Autodesk Inventor part; units mm, degrees
ref_plane "Work Plane1" through (0, 0, -7) normal (0, 0, -1) x (-1, 0, 0)
ref_plane "YZ Plane" through (0, 0, 0) normal (1, 0, 0) x (0, 1, 0)
ref_plane "XZ Plane" through (0, 0, 0) normal (0, 1, 0) x (-1, 0, 0)
sketch "Sketch1" plane through (0, 0, 0) normal (0, 0, 1) x (1, 0, 0)
  circle A0 centre (0, 0) radius 2.5
  circle A1 centre (20, 0) radius 2.5
  line L0 (7, 10) -> (20, 10)
  line L1 (7, -10) -> (20, -10)
  arc A2 (20, -10) -> (20, 10) centre (20, 0) ccw
  line L2 (7, 10) -> (7, 8)
  line L3 (7, -10) -> (7, -8)
  line L4 (7, 8) -> (0, 8)
  line L5 (7, -8) -> (0, -8)
  arc A3 (0, 8) -> (0, -8) centre (0, 0) ccw
  dimension "d0" = 5
  dimension "d1" = 20
  dimension "d2" = 10
  dimension "d3" = 2
  dimension "d4" = 13
extrude "Extrusion1" add sketch "Sketch1" along normal blind 4
sketch "Sketch2" plane through (0, 0, 4) normal (0, 0, 1) x (1, 0, 0)
  circle A0 centre (0, 0) radius 2.5
  line L0 (7, 8) -> (0, 8)
  arc A1 (0, 8) -> (0, -8) centre (0, 0) ccw
  line L1 (0, -8) -> (7, -8)
  line L2 (7, -10) -> (20, -10)
  line L3 (7, 8) -> (7, -8)
  line L4 (7, -8) -> (0, -8)
  line L5 (7, 8) -> (0, 8)
  arc A2 (0, 8) -> (0, -8) centre (0, 0) ccw
extrude "Extrusion2" cut sketch "Sketch2" against normal blind 2
sketch "Sketch3" plane through (0, 0, 0) normal (0, 0, -1) x (-1, 0, 0)
  circle A0 centre (-20, 0) radius 2.5
  circle A1 centre (0, 0) radius 2.5
  line L0 (-7, 10) -> (-20, 10)
  arc A2 (-20, 10) -> (-20, -10) centre (-20, 0) ccw
  line L1 (-20, -10) -> (-7, -10)
  line L2 (-7, 8) -> (-7, 10)
  line L3 (-19, 10) -> (-19, 8)
  line L4 (-19, 8) -> (-11, 8)
  line L5 (-11, 8) -> (-11, -8)
  line L6 (-11, -8) -> (-19, -8)
  line L7 (-19, -8) -> (-19, -10)
  point P0 (-7, -8)
  dimension "d9" = 1
  dimension "d10" = 11
extrude "Extrusion3" cut sketch "Sketch3" against normal blind 2 contours L3 L4 L5 L6 L7 L1 A2 L0
sketch "Sketch4" plane through (0, 0, 4) normal (0, 0, 1) x (1, 0, 0)
  line L0 (7, 10) -> (7, -10)
  circle A0 centre (0, 0) radius 2.5
  arc A1 (7, -8.4853) -> (7, 8.4853) centre (0, 0) ccw
  dimension "d15" = 11
extrude "Extrusion4" cut sketch "Sketch4" against normal blind 2 contours A1 L0
sketch "Sketch5" plane through (0, 0, 0) normal (0, 0, -1) x (-1, 0, 0)
  line L0 (0, 8) -> (-7, 8)
  line L1 (-7, 10) -> (0, 10)
  line L2 (0, 10) -> (0, 8)
  line L3 (0, 8) -> (-7, 8)
  line L4 (-7, 8) -> (-7, 10)
  arc A0 (0, -8) -> (0, 8) centre (0, 0) ccw
extrude "Extrusion5" add sketch "Sketch5" against normal blind 2
sketch "Sketch6" plane through (0, 0, 0) normal (0, 0, -1) x (-1, 0, 0)
  line L0 (0, 10) -> (-19, 10)
  line L1 (-19, 8) -> (-20, 8)
  line L2 (-20, 8) -> (-20, 10)
  line L3 (-20, 10) -> (-19, 10)
  line L4 (-19, 10) -> (-19, 8)
  circle A0 centre (-20, 0) radius 2.5
extrude "Extrusion6" add sketch "Sketch6" against normal blind 2 contours L1 L2 L3 L4
sketch "Sketch7" plane through (0, 0, 0) normal (0, 0, -1) x (-1, 0, 0)
  line L0 (-19, -8) -> (-19, -10)
  line L1 (-11, -8) -> (-19, -8)
  line L2 (-17.4006, -8) -> (-19, -9.162)
  line L3 (-17.4006, -8) -> (-26.8052, 4.9443) construction
  line L4 (-26.8052, 4.9443) -> (-28.4046, 3.7823) construction
  line L5 (-28.4046, 3.7823) -> (-19, -9.162) construction
  circle A0 centre (-20, 0) radius 2.5
  line L6 (-17.4006, -8) -> (-19, -8)
  line L7 (-19, -8) -> (-19, -9.162)
  dimension "d21" = 16
  dimension "d22" = 8
  dimension "d23" = 36
extrude "Extrusion7" cut sketch "Sketch7" against normal blind 2 contours L1 L2 L0
sketch "Sketch9" plane through (0, 0, 2) normal (0, 0, 1) x (1, 0, 0)
  circle A0 centre (0, 0) radius 2.5
  arc A1 (11, 0) -> (7, 8.4853) centre (0, 0) ccw
  circle A2 centre (0, 0) radius 2.5
extrude "Extrusion8" add sketch "Sketch9" along normal mid plane 4
fillet "Fillet1" radius 0.5 1 edges at (-2.5, 0, 4)
sketch "Sketch10" plane through (0, 0, 0) normal (0, 0, -1) x (-1, 0, 0)
  arc A0 (0, -8) -> (0, 8) centre (0, 0) ccw
  line L0 (0, 10) -> (-20, 10)
  line L1 (4.7023, 6.4721) -> (11.1744, 1.7699)
  line L2 (11.1744, 1.7699) -> (6.4721, -4.7023)
  dimension "d30" = 144
extrude "Extrusion9" add sketch "Sketch10" against normal blind 2
fillet "Fillet2" radius 6 1 edges at (-11.1744, 1.7699, 1)
ref_plane "Work Plane1" through (0, 0, -7) normal (0, 0, -1) x (-1, 0, 0)
mirror "Mirror1" about plane through (0, 0, -7) normal (0, 0, -1)
sketch "Sketch11" plane through (0, 0, 0) normal (0, 0, -1) x (-1, 0, 0)
  arc A0 (4.7023, 6.4721) -> (0, 8) centre (0, 0) ccw
  line L0 (0, 8) -> (0, 10)
  line L1 (0, 10) -> (-20, 10)
  line L2 (-20, 10) -> (-20, 8)
  line L3 (-20, 8) -> (-11, 8)
  line L4 (-11, -8) -> (-17.4006, -8)
  line L5 (-17.4006, -8) -> (-19, -9.162)
  line L6 (-19, -9.162) -> (-19, -10)
  line L7 (-19, -10) -> (-7, -10)
  line L8 (-7, -10) -> (-7, -8)
  line L9 (-7, -8) -> (0, -8)
  line L10 (-11, -8) -> (-7, -8)
  line L11 (-11, 8) -> (0, 8)
extrude "Extrusion10" add sketch "Sketch11" along normal blind 14
properties part number "cable_chain_22" material "ABS Plastic"
Source: CAD feature listing. Evaluate the final solid. Frame: model axes, mm. A direction names the side the tool comes from. Coordinates: 2 decimals unless noted, no trailing zeros. Loops run counter-clockwise (first coordinate to the right, second up) from the corner with the lowest first, then second, coordinate; pieces in that order, holes last. Notation, with made-up numbers: (31.5, 34) -> (38.5, 34) arc R28 cw to (38.5, 70) -> close; hole circle Ø11 at (32.25, 44.5). An arc over 180 degrees is marked (long way). Answer in a Markdown table with one row per item. Add a question column.
Q1. Ray query, line 1 along Y through (x, z) = (12.5, -5.5); line 2 along Y through (x, z) = (20, 2.5); line 3 along Z through (x, y) = (17, 3.25). Return the intervals inside material, ascending.
Q2. Section B-B on z = -12. Return the cut outline in (x, y), and give its area (3 significant figures).
Q3. Section A-A on z = 2.75. Return the cut outline in (x, y).
Q4. Pull-direction query (Z, two-part tool) for faces 6 (the face through (10, 8, -7)), 7 (the face through (18.189, -8.573, -6.874)), 8 (the face through (10, 10, -7)), 9 (the face through (3, 1, 2)); classes: pulls with the +Z half, pulls with the -Z half, needs draft (parallel to the pull), parting line crosses it, or undercut.
Q5. Section C-C on x = 22. Return the cut outline in (y, z), and give its area (3 significant figures).
Q6. Contact query for flat-ended pins moving along their axis: pin 1 Ø6 at (x, y) = (9.5, 4.5) entering from -Z; pin 2 Ø1.6 at (x, z) = (3.5, 0.5) entering from -Y; pin 3 Ø1.7 at (y, z) = (9, -17) entering from -X; pin 4 Ø1.6 at (y, z) = (9.5, -4.5) entering from +X. Output: stop coordinate, or through.
Q7. Reachability of faces 1 (the face through (11, 0, -15)), 2 (the face through (1, 0, -14)), 3 (the face through (-5.5, 5.893, 0.986)), 4 (the face through (7, 9, 3)), 5 (the face through (3, 1, -16)) from +Z, -Z, +X, -X, +Y, -Y: full face, straight path, thin tool, end or side. Return the list, or none.
Q8. Section D-D on y = -6.5. Return the cut outline in (x, z), and give its area (3 significant figures).
Computed values:
| question | item | result |
|---|---|---|
| 1 | line 1 | y = -10 to -8, 8 to 10 |
| 1 | line 2 | y = -10 to -2.5, 2.5 to 10 |
| 1 | line 3 | z = -18 to -16, 2 to 4 |
| 2 | outline | (0, 8) -> (20, 8) -> (20, 10) -> (0, 10) -> close; (7, -10) -> (19, -10) -> (19, -9.16) -> (17.4, -8) -> (7, -8) -> close |
| 2 | area | 63.1 mm^2 |
| 3 | outline | circle Ø5 at (0, 0); (7, -10) -> (20, -10) arc R10 ccw to (20, 10) -> (7, 10) -> (7, 8.49) arc R11 cw to (7, -8.49) -> close; hole circle Ø5 at (20, 0) |
| 4 | face 6 | undercut |
| 4 | face 7 | undercut |
| 4 | face 8 | needs draft |
| 4 | face 9 | pulls with the +Z half |
| 5 | outline | (-9.8, -18) -> (-1.5, -18) -> (-1.5, -16) -> (-9.8, -16) -> close; (-9.8, 2) -> (-1.5, 2) -> (-1.5, 4) -> (-9.8, 4) -> close; (1.5, -18) -> (9.8, -18) -> (9.8, -16) -> (1.5, -16) -> close; (1.5, 2) -> (9.8, 2) -> (9.8, 4) -> (1.5, 4) -> close |
| 5 | area | 66.4 mm^2 |
| 6 | pin 1 | stops at z = -18 |
| 6 | pin 2 | stops at y = -8 |
| 6 | pin 3 | stops at x = 7 |
| 6 | pin 4 | stops at x = 20 |
| 7 | face 1 | +X |
| 7 | face 2 | +X, -X |
| 7 | face 3 | +Z, -Z, -X, +Y |
| 7 | face 4 | +Z, -X, +Y, -Y |
| 7 | face 5 | -Z |
| 8 | outline | (-4.66, -16) -> (8.87, -16) -> (8.87, -18) -> (27.6, -18) -> (27.6, -16) -> (11, -16) -> (11, -14) -> (-4.66, -14) -> close; (-4.66, 0) -> (11, 0) -> (11, 2) -> (27.6, 2) -> (27.6, 4) -> (8.87, 4) -> (8.87, 2) -> (-4.66, 2) -> close |
| 8 | area | 138 mm^2 |
